Source: three-view drawing plus pictorial views. Frame: mm from the lowest corner of the part. A direction names the side the tool comes from. Give positions to 0.01 mm unless a question says otherwise; leave off trailing zeros. Order: outer loops, then holes, each group sorted by start corner. A loop starts at its lowest first (then second) coordinate and runs counter-clockwise, first axis right, second up. Notation, with made-up numbers: M 11.25,49.25 L 32.25,49.25 A21 ccw 32.25,56.25 Z; hole C -33,81 d11. An arc over 180 degrees is marked long. Use CSV: the item, a comma, the result in double quotes. Start each with the question number.
Item 1: Access query for the marked faces 4, 5 and 6. Directions: +Z, -Z, +X, -X, +Y, -Y. A direction counts if a zero-diameter tool reaches every point of the face in a straight line with its end or side. Return the directions, or none.
Item 2: Section query C-C on z = 4.75. Return loops of the section in (x, y) (1 decimal).
Item 3: First-contact query: pin 1 (3 mm diameter, centred on x = 31.5, y = 4.5, fed in from -Z); pin 2 (10 mm diameter, centred on y = 6, z = 12, fed in from -X); pin 3 (3 mm diameter, centred on x = 31.5, y = 3.5, fed in from +Z); pin 4 (10 mm diameter, centred on x = 4, y = 5, fed in from +Z). Flat tips, straight axial feed; report the tip coordinate or a pass-through.
Item 4: Ray query, probe 1 along X at (y, z) = (4.25, 17.5) (1 decimal); probe 2 along Y at (x, z) = (4, 10.25) (1 decimal); probe 3 along Z at (x, y) = (34, 11.25) (1 decimal). Return the intervals inside material, ascending. Write a range as from..to.
Item 5: Pull-direction query (Y, two-part tool) for the marked faces 1, 2 and 3; classes: +Y half, -Y half, draft (parallel to the pull), parting line (faces both ways), or undercut.
Item 6: Section query A-A on y = 9. Return loops of the section in (x, z) (1 decimal).
Item 7: Section query B-B on z = 13.25. Return loops of the section in (x, y) (1 decimal).
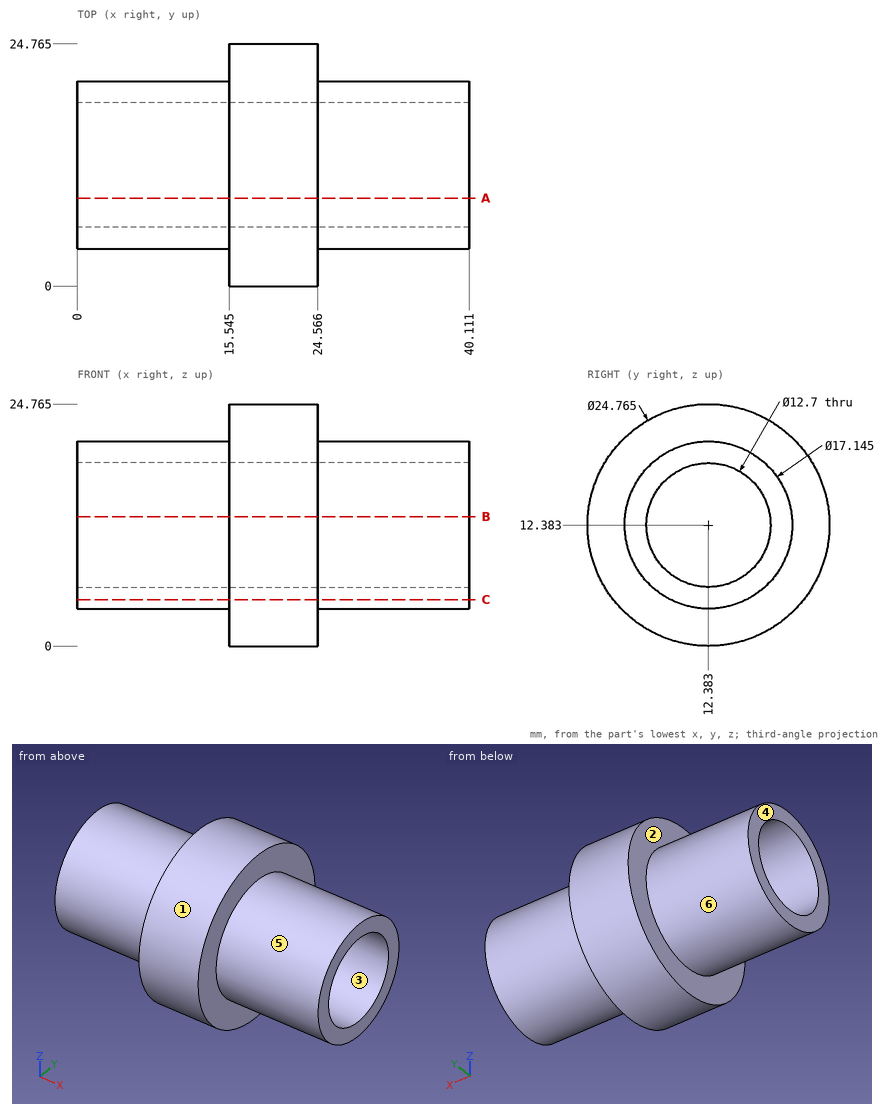
Verdict:
1,face 4,"+Z, -Z, -X, +Y, -Y"
1,face 5,"+X"
1,face 6,"-X"
2,outline,"M 0,8.5 L 15.5,8.5 L 15.5,2.6 L 24.6,2.6 L 24.6,8.5 L 40.1,8.5 L 40.1,16.3 L 24.6,16.3 L 24.6,22.1 L 15.5,22.1 L 15.5,16.3 L 0,16.3 Z"
3,pin 1,"z = 6.66"
3,pin 2,"x = 0"
3,pin 3,"z = 16.74"
3,pin 4,"z = 20.62"
4,probe 1,"15.5..24.6"
4,probe 2,"4.1..6.4, 18.4..20.7"
4,probe 3,"3.9..6.1, 18.6..20.9"
5,face 1,"parting line"
5,face 2,"draft"
5,face 3,"undercut"
6,outline,"M 0,4.5 L 15.5,4.5 L 15.5,0.5 L 24.6,0.5 L 24.6,4.5 L 40.1,4.5 L 40.1,7 L 0,7 Z; M 0,17.8 L 40.1,17.8 L 40.1,20.3 L 24.6,20.3 L 24.6,24.3 L 15.5,24.3 L 15.5,20.3 L 0,20.3 Z"
7,outline,"M 0,3.9 L 15.5,3.9 L 15.5,0 L 24.6,0 L 24.6,3.9 L 40.1,3.9 L 40.1,6.1 L 0,6.1 Z; M 0,18.7 L 40.1,18.7 L 40.1,20.9 L 24.6,20.9 L 24.6,24.7 L 15.5,24.7 L 15.5,20.9 L 0,20.9 Z"
